Geometry check sheet. Reference: the model listing, model coordinates, mm. Face numbers are marked on the shaded views. Round coordinates to 2 decimals unless told otherwise and drop trailing zeros. Write each loop counter-clockwise with the first axis right and the second up, starting at its lowest first coordinate (ties: lowest second). Pieces come first, ordered by that corner, then holes. Notation, with made-up numbers: (63.25, 62.25) -> (118.25, 62.25) arc R30 ccw to (118.25, 98.25) -> close; hole circle Ø6 at (29, 67). An arc over 180 degrees is marked (long way). Use a Markdown table: item, result.
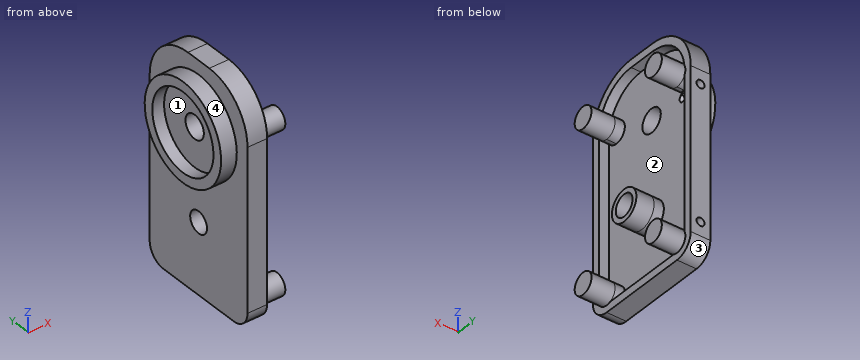
```python
from build123d import *

# Parameters (mm, degrees)
SKETCH1_W                    = 58
SKETCH1_H                    = 32
SKETCH1_R                    = 2.75
BOSS_EXTRUDE1_DEPTH          = 5
SKETCH2_R                    = 4
SKETCH2_R_2                  = 2.75
BOSS_EXTRUDE2_DEPTH          = 4.5
FILLET1_R                    = 4.5
FILLET2_R                    = 12.5
SKETCH4_R                    = 2.75
BOSS_EXTRUDE3_DEPTH          = 6
SKETCH8_R                    = 12.5
BOSS_EXTRUDE4_DEPTH          = 4
SKETCH9_R                    = 10
CUT_EXTRUDE2_DEPTH           = 3
SKETCH10_R                   = 3
CUT_EXTRUDE3_DEPTH           = 13
SKETCH3_R                    = 4
CUT_EXTRUDE1_DEPTH           = 2.5
M2_5X0_45_TAPPED_HOLE1_D     = 2.05
M2_5X0_45_TAPPED_HOLE1_DEPTH = 6.35
M2_5X0_45_TAPPED_HOLE1_TIP   = 0.615882135


with BuildPart() as part:
    # Sketch1 → Boss-Extrude1 (new body)
    with BuildSketch(Plane(origin=(0, 0, 0), x_dir=(0, 0, -1), z_dir=(1, 0, 0))):
        Rectangle(SKETCH1_W, SKETCH1_H)
        with Locations((11, 0)):
            Circle(SKETCH1_R, mode=Mode.SUBTRACT)
    extrude(amount=BOSS_EXTRUDE1_DEPTH)

    # Sketch2 → Boss-Extrude2 (add)
    with BuildSketch(Plane(origin=(5, 0, 0), x_dir=(0, 0, -1), z_dir=(1, 0, 0))):
        with Locations((11, 0)):
            Circle(SKETCH2_R)
        with Locations((11, 0)):
            Circle(SKETCH2_R_2, mode=Mode.SUBTRACT)
    extrude(amount=BOSS_EXTRUDE2_DEPTH)

    # Fillet1
    fillet1_edges = [part.edges().sort_by_distance(p)[0] for p in [
        (2.5, 16, -29),
        (2.5, -16, -29),
    ]]
    fillet(fillet1_edges, radius=FILLET1_R)

    # Fillet2
    fillet2_edges = [part.edges().sort_by_distance(p)[0] for p in [
        (2.5, -16, 29),
        (2.5, 16, 29),
    ]]
    fillet(fillet2_edges, radius=FILLET2_R)

    # Sketch4 → Boss-Extrude3 (add)
    with BuildSketch(Plane(origin=(5, 0, 0), x_dir=(0, 0, -1), z_dir=(1, 0, 0))):
        with Locations((24.5, 11.5)):
            Circle(SKETCH4_R)
        with Locations((24.5, -11.5)):
            Circle(SKETCH4_R)
        with Locations((-16.5, 11.5)):
            Circle(SKETCH4_R)
        with Locations((-16.5, -11.5)):
            Circle(SKETCH4_R)
    extrude(amount=BOSS_EXTRUDE3_DEPTH)

    # Sketch8 → Boss-Extrude4 (add)
    with BuildSketch(Plane.ZY):
        with Locations((13, 0)):
            Circle(SKETCH8_R)
    extrude(amount=BOSS_EXTRUDE4_DEPTH)

    # Sketch9 → Cut-Extrude2 (cut)
    with BuildSketch(Plane.ZY.offset(4)):
        with Locations((13, 0)):
            Circle(SKETCH9_R)
    extrude(amount=-CUT_EXTRUDE2_DEPTH, mode=Mode.SUBTRACT)

    # Sketch10 → Cut-Extrude3 (cut, through all)
    with BuildSketch(Plane.ZY.offset(1)):
        with Locations((13, 0)):
            Circle(SKETCH10_R)
    extrude(amount=-CUT_EXTRUDE3_DEPTH, mode=Mode.SUBTRACT)

    # Sketch3 → Cut-Extrude1 (cut)
    with BuildSketch(Plane(origin=(5, 0, 0), x_dir=(0, 0, -1), z_dir=(1, 0, 0))):
        with BuildLine():
            ThreePointArc((-17.809934015, 13.91796875), (-24.374144625, 10.446066975), (-27, 3.5))
            Line((-27, 3.5), (-27, -3.5))
            ThreePointArc((-27, -3.5), (-24.374144625, -10.446066975), (-17.809934015, -13.91796875))
            ThreePointArc((-17.809934015, -13.91796875), (-17.907156967, -9.13728773), (-13.75, -11.5))
            ThreePointArc((-13.75, -11.5), (-14.185586382, -12.98525742), (-15.354356076, -14))
            Line((-15.354356076, -14), (23.354356076, -14))
            ThreePointArc((23.354356076, -14), (22.555456352, -9.555456352), (27, -10.354356076))
            Line((27, -10.354356076), (27, 10.354356076))
            ThreePointArc((27, 10.354356076), (22.555456352, 9.555456352), (23.354356076, 14))
            Line((23.354356076, 14), (-15.354356076, 14))
            ThreePointArc((-15.354356076, 14), (-14.185586382, 12.98525742), (-13.75, 11.5))
            ThreePointArc((-13.75, 11.5), (-17.907156967, 9.13728773), (-17.809934015, 13.91796875))
        make_face()
        with Locations((11, 0)):
            Circle(SKETCH3_R, mode=Mode.SUBTRACT)
    extrude(amount=-CUT_EXTRUDE1_DEPTH, mode=Mode.SUBTRACT)

    # M2.5x0.45 Tapped Hole1
    with Locations(Plane(origin=(0, 16, 0), x_dir=(1, 0, 0), z_dir=(0, 1, 0))):
        with Locations((2.5, 21), (2.5, -13)):
            Hole(M2_5X0_45_TAPPED_HOLE1_D / 2, depth=M2_5X0_45_TAPPED_HOLE1_DEPTH)
            with Locations((0, 0, -(M2_5X0_45_TAPPED_HOLE1_DEPTH + M2_5X0_45_TAPPED_HOLE1_TIP / 2))):  # 118° drill point
                Cone(0, M2_5X0_45_TAPPED_HOLE1_D / 2, M2_5X0_45_TAPPED_HOLE1_TIP, mode=Mode.SUBTRACT)


solid = part.part
```
(1) Section check D-D on y = -1.5. Record the cut outline in (x, z).
A:
| item | result |
|---|---|
| outline | (-4, 0.59) -> (0, 0.59) -> (0, -8.7) -> (9.5, -8.7) -> (9.5, -7.29) -> (2.5, -7.29) -> (2.5, 10.4) -> (-1, 10.4) -> (-1, 3.11) -> (-4, 3.11) -> close; (-4, 22.89) -> (-1, 22.89) -> (-1, 15.6) -> (2.5, 15.6) -> (2.5, 27) -> (5, 27) -> (5, 29) -> (0, 29) -> (0, 25.41) -> (-4, 25.41) -> close; (0, -29) -> (5, -29) -> (5, -27) -> (2.5, -27) -> (2.5, -14.71) -> (9.5, -14.71) -> (9.5, -13.3) -> (0, -13.3) -> close |
(2) Thickness scan on line 1 (Y direction, x = -2, z = 12.5); line 2 (X direction, y = 12, z = 13) (3 decimals); line 3 (X direction, y = -10.5, z = -7). Record the ranges inside material, lowest first.
A:
| item | result |
|---|---|
| line 1 | y = -12.49 to -9.99, 9.99 to 12.49 |
| line 2 | x = -4 to 1.475 |
| line 3 | x = 0 to 2.5 |
(3) Section check C-C on z = 13. Record the cut outline in (x, y) (3 decimals), plus the area to 3 significant figures.
A:
| item | result |
|---|---|
| outline | (-4, -12.5) -> (0, -12.5) -> (0, -16) -> (5, -16) -> (5, -14) -> (2.5, -14) -> (2.5, -3) -> (-1, -3) -> (-1, -10) -> (-4, -10) -> close; (-4, 10) -> (-1, 10) -> (-1, 3) -> (2.5, 3) -> (2.5, 9.034) -> (1.475, 9.65) -> (1.475, 16) -> (0, 16) -> (0, 12.5) -> (-4, 12.5) -> close; (3.525, 14) -> (5, 14) -> (5, 16) -> (3.525, 16) -> close |
| area | 100 mm2 |
(4) Release check for a two-part mould opening along Y. For the marked faces 1, 2, 3 and 4 record: +Y half, -Y half, draft (parallel to the pull), parting line (faces both ways), or undercut.
A:
| item | result |
|---|---|
| face 1 | undercut |
| face 2 | undercut |
| face 3 | +Y half |
| face 4 | parting line |
(5) Section check B-B on z = -11. Record the cut outline in (x, y), plus the area to 4 significant figures.
A:
| item | result |
|---|---|
| outline | (0, -16) -> (5, -16) -> (5, -14) -> (2.5, -14) -> (2.5, -4) -> (9.5, -4) -> (9.5, -2.75) -> (0, -2.75) -> close; (0, 2.75) -> (9.5, 2.75) -> (9.5, 4) -> (2.5, 4) -> (2.5, 14) -> (5, 14) -> (5, 16) -> (0, 16) -> close |
| area | 93.75 mm2 |
(6) Gauge pin test, flat ends, axial feed: pin 1 Ø14 at (y, z) = (3, 3.5) entering from +X; pin 2 Ø9.5 at (y, z) = (0, 13) entering from -X; pin 3 Ø6 at (x, y) = (7.5, -5.5) entering from +Z. Record the tip position at first contact, or that the pin passes through.
A:
| item | result |
|---|---|
| pin 1 | stops at x = 2.5 |
| pin 2 | stops at x = -1 |
| pin 3 | stops at z = 29 |
(7) Section check A-A on x = 6.25. Record the cut outline in (y, z), plus the area to 3 significant figures.
A:
| item | result |
|---|---|
| outline | circle Ø5.5 at (-11.5, -24.5); circle Ø5.5 at (-11.5, 16.5); circle Ø8 at (0, -11); circle Ø5.5 at (11.5, -24.5); circle Ø5.5 at (11.5, 16.5); hole circle Ø5.5 at (0, -11) |
| area | 122 mm2 |
